Geometry check sheet. Reference: the model listing, model coordinates, mm. A direction names the side the tool comes from. Coordinates: 2 decimals unless noted, no trailing zeros. Loops run counter-clockwise (first coordinate to the right, second up) from the corner with the lowest first, then second, coordinate; pieces in that order, holes last. Notation, with made-up numbers: (47, -30.5) - (70, -30.5) arc R17 ccw to (70, -11.5) - close; hole circle Ø5 at (66, 45.25). An arc over 180 degrees is marked (long way). Write each question's results on one line, items separated by ' | '. Start each with the question number.
(1) Sectioned sample at A-A (y = 2.5). Enter the section's corners in (x, z), plus the area to 3 significant figures.
(2) Sectioned sample at C-C (z = -111). Enter the section's corners in (x, y).
(3) Access from +Z, -Z, +X, -X, +Y, -Y to the whole of each face (thin tool, end or side, straight path). Record for faces 1 (the face through (51.3, 2.54, -81.57)), 2 (the face through (58, -5, -69)).
(4) Go/stop test with flat-tipped pins: pin 1 Ø3 at (y, z) = (0.5, -67.5) entering from +X; pin 2 Ø5 at (x, z) = (106.5, -111) entering from +Y; pin 3 Ø3 at (y, z) = (2, -63) entering from -X. Record where each tip stops, or that it passes through.
(5) Sectioned sample at B-B (x = 99). Enter the section's corners in (y, z), plus the area to 3 significant figures.
(6) Sectioned sample at D-D (x = 120). Enter the section's corners in (y, z).
(7) Mould release check, pull along Z, two halves, no side actions. Record for faces 3 (the face through (56.425, 2.465, -72.981)), 4 (the face through (35.92, -0.07, -107.325)), 5 (the face through (149.825, -1.181, -86.299)), 6 (the face through (48, 5, -105)): pulls with the +Z half, pulls with the -Z half, needs draft (parallel to the pull), parting line crosses it, or undercut.
(8) Material ranges on probe 1 along X at (y, z) = (4, -66); probe 2 along X at (y, z) = (2.75, -69.5); probe 3 along X at (y, z) = (3.25, -45), recorded low to high.
from build123d import *


with BuildPart() as part:
    # Sweep1: sweep along a path in Sketch2
    with BuildLine(Plane(origin=(0, 0, 0), x_dir=(1, 0, 0), z_dir=(0, 1, 0))) as sweep1_path:
        ThreePointArc((0, 0), (50, 86.602540378), (150, 86.602540378))
    # Sketch1 → Sweep1 (sweep)
    with BuildSketch(Plane.XY):
        Polygon((25, -5), (-25, -5), (-25, 5), (-15, 5), (-15, 0), (-5, 0), (-5, 5), (5, 5), (5, 0), (15, 0), (15, 5), (25, 5), align=None)
    sweep(path=sweep1_path.line)


solid = part.part
Outcome:
1) outline: (-25, 0) arc R125 ccw to (162.5, -108.25) - (157.5, -99.59) arc R115 cw to (-15, 0) - close; (-5, 0) arc R105 ccw to (152.5, -90.93) - (147.5, -82.27) arc R95 cw to (5, 0) - close; (15, 0) arc R85 ccw to (142.5, -73.61) - (137.5, -64.95) arc R75 cw to (25, 0) - close | area: 6,280 mm2
2) outline: (42.52, -5) - (157.48, -5) - (157.48, 5) - (130.07, 5) - (130.07, 0) - (69.93, 0) - (69.93, 5) - (42.52, 5) - close
3) face 1: +Y | face 2: +Z, -Z, +X, -X, -Y
4) pin 1: stops at x = 139.84 | pin 2: stops at y = 0 | pin 3: stops at x = -8.82
5) outline: (-5, -125) - (5, -125) - (5, -115) - (0, -115) - (0, -105) - (5, -105) - (5, -94.99) - (0, -94.99) - (0, -84.99) - (5, -84.99) - (5, -74.99) - (-5, -74.99) - close | area: 400 mm2
6) outline: (-5, -123.39) - (5, -123.39) - (5, -113.25) - (0, -113.25) - (0, -103.08) - (5, -103.08) - (5, -92.87) - (0, -92.87) - (0, -82.61) - (5, -82.61) - (5, -72.28) - (-5, -72.28) - close
7) face 3: undercut | face 4: pulls with the -Z half | face 5: pulls with the +Z half | face 6: needs draft
8) probe 1: x = -6.16 to 5.82, 18.34 to 31.67, 46.44 to 64.38, 135.62 to 138.11 | probe 2: x = -3.9 to 8.38, 21.29 to 35.23, 51.06 to 71.81, 128.19 to 140.13 | probe 3: x = -16.62 to -5.83, 5.13 to 16.33, 27.89 to 40
